For this review, use the dimensioned drawing (mm, ordinates from the lowest corner) and the shaded views. Round coordinates to 2 decimals unless told otherwise and drop trailing zeros. Write each loop counter-clockwise with the first axis right and the second up, starting at its lowest first coordinate (ties: lowest second). Pieces come first, ordered by that corner, then holes.
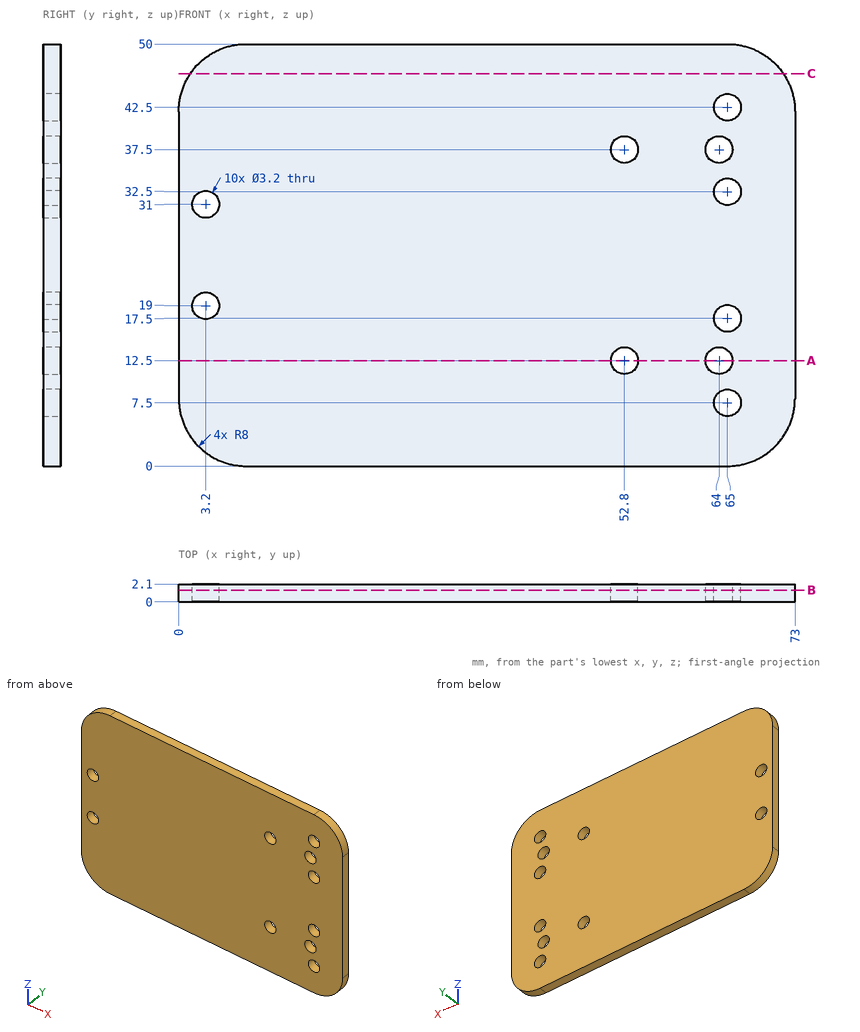
(1) We need section A-A, the plane z = 12.5. Give the boundary of the cut face in (x, y), and give its area (3 significant figures).
Geometry check:
outline: (0, 0) - (51.2, 0) - (51.2, 2.1) - (0, 2.1) - close; (54.4, 0) - (62.4, 0) - (62.4, 2.1) - (54.4, 2.1) - close; (65.6, 0) - (73, 0) - (73, 2.1) - (65.6, 2.1) - close
area: 140 mm2
(2) For pin 1 Ø2.5 at (x, z) = (52.8, 12.5) entering from -Y, flat-tipped, find the tip position at first contact; note if it passes through.
Geometry check:
pin 1: passes through
(3) We need section C-C, the plane z = 46.5. Give the boundary of the cut face in (x, y), and give its area (3 significant figures).
Geometry check:
outline: (1.39, 0) - (71.61, 0) - (71.61, 2.1) - (1.39, 2.1) - close
area: 147 mm2
(4) For line 1 along X through (y, z) = (1, 37.5); line 2 along X through (y, z) = (1.2, 7.5); line 3 along X through (y, z) = (0.85, 37), list the stretches that pass through material, from the lowest coordinate up.
Geometry check:
line 1: x = 0 to 51.2, 54.4 to 62.4, 65.6 to 73
line 2: x = 0.02 to 63.4, 66.6 to 72.98
line 3: x = 0 to 51.28, 54.32 to 62.48, 65.52 to 73
(5) We need section B-B, the plane y = 1.4. State how many separate pieces and enclosed holes the cut face has, and give its area (3 significant figures).
Geometry check:
separate pieces: 1
enclosed holes: 10
area: 3,510 mm2
